Geometry: final body of the model. Coordinates: model frame, mm. A direction names the side the tool comes from. Round coordinates to 2 decimals unless told otherwise and drop trailing zeros. Loops run counter-clockwise (first coordinate to the right, second up) from the corner with the lowest first, then second, coordinate; pieces in that order, holes last. Notation, with made-up numbers: (46.5, 17.25) - (58.5, 17.25) arc R28 ccw to (58.5, 44.25) - close; hole circle Ø2 at (-21, 72). An arc over 180 degrees is marked (long way). Answer as CSV lines item,"result".
from build123d import *

# Parameters (mm, degrees)
SKETCH_1_W      = 18
SKETCH_1_H      = 18
EXTRUDE_1_DEPTH = 1.6
EXTRUDE_START   = 1.6
EXTRUDE_2_DEPTH = 1.9
SKETCH_3_W      = 16.5
SKETCH_3_H      = 16.5
EXTRUDE_3_DEPTH = 1


with BuildPart() as part:
    # 草图1 → 凸台-拉伸1 (new body)
    with BuildSketch(Plane(origin=(0, 0, 0), x_dir=(1, 0, 0), z_dir=(0, 1, 0))):
        Rectangle(SKETCH_1_W, SKETCH_1_H)
    extrude(amount=EXTRUDE_1_DEPTH)

    # 草图2 → 凸台-拉伸2 (add)
    with BuildSketch(Plane(origin=(0, 0, 0), x_dir=(1, 0, 0), z_dir=(0, 1, 0)).offset(EXTRUDE_START)):
        with BuildLine():
            Line((-6.5, 8), (6.5, 8))
            ThreePointArc((6.5, 8), (7.560660172, 7.560660172), (8, 6.5))
            Line((8, 6.5), (8, -6.5))
            ThreePointArc((8, -6.5), (7.560660172, -7.560660172), (6.5, -8))
            Line((6.5, -8), (-6.5, -8))
            ThreePointArc((-6.5, -8), (-7.560660172, -7.560660172), (-8, -6.5))
            Line((-8, -6.5), (-8, 6.5))
            ThreePointArc((-8, 6.5), (-7.560660172, 7.560660172), (-6.5, 8))
        make_face()
    extrude(amount=EXTRUDE_2_DEPTH)

    # 草图3 → 凸台-拉伸3 (add)
    with BuildSketch(Plane(origin=(0, 0, 0), x_dir=(1, 0, 0), z_dir=(0, 1, 0))):
        Rectangle(SKETCH_3_W, SKETCH_3_H)
    extrude(amount=-EXTRUDE_3_DEPTH)


solid = part.part
(1) Section A-A (z = 2.5). Output: boundary loops of the cut face in (x, y).
Findings below:
outline,"(-9, 0) - (-8.25, 0) - (-8.25, -1) - (8.25, -1) - (8.25, 0) - (9, 0) - (9, 1.6) - (8, 1.6) - (8, 3.5) - (-8, 3.5) - (-8, 1.6) - (-9, 1.6) - close"
(2) Section C-C (x = 0.5). Output: boundary loops of the cut face in (y, z), and give its area (3 significant figures).
Findings below:
outline,"(-1, -8.25) - (0, -8.25) - (0, -9) - (1.6, -9) - (1.6, -8) - (3.5, -8) - (3.5, 8) - (1.6, 8) - (1.6, 9) - (0, 9) - (0, 8.25) - (-1, 8.25) - close"
area,"75.7 mm2"
(3) Access query for faces 1 (the face through (0, 3, 8)), 2 (the face through (7.55, 2.54, -7.57)), 3 (the face through (8, 3, 0)), 4 (the face through (7.57, 2.54, 7.55)), 5 (the face through (0, 3, -8)). Directions: +Z, -Z, +X, -X, +Y, -Y. A direction counts if a zero-diameter tool reaches every point of the face in a straight line with its end or side. Return the directions, or none.
Findings below:
face 1,"+Z, +X, -X, +Y"
face 2,"-Z, +X, +Y"
face 3,"+Z, -Z, +X, +Y"
face 4,"+Z, +X, +Y"
face 5,"-Z, +X, -X, +Y"
(4) Material intervals for line 1 along X through (y, z) = (-0.65, -0.5); line 2 along X through (y, z) = (2.65, 0.75), sorted ascending.
Findings below:
line 1,"-8.25 to 8.25"
line 2,"-8 to 8"
(5) Section B-B (y = 3). Output: boundary loops of the cut face in (x, z).
Findings below:
outline,"(-8, -6.5) arc R1.5 ccw to (-6.5, -8) - (6.5, -8) arc R1.5 ccw to (8, -6.5) - (8, 6.5) arc R1.5 ccw to (6.5, 8) - (-6.5, 8) arc R1.5 ccw to (-8, 6.5) - close"
(6) Pin query (flat end, axial travel): P1, Ø0.6, axis at y = 2.5, z = -2, coming from the -X side; P2, Ø0.8, axis at y = -0.5, z = 1, coming from the -X side; P3, Ø0.6, axis at x = -1.5, y = 2.5, coming from the +Z side. Return the tip coordinate at first contact, or that it passes through.
Findings below:
P1,"x = -8"
P2,"x = -8.25"
P3,"z = 8"
